CAD build for the part. Positions are in the model's coordinates, mm. Round coordinates to 2 decimals unless told otherwise and drop trailing zeros. Order: outer loops, then holes, each group sorted by start corner. A loop starts at its lowest first (then second) coordinate and runs counter-clockwise, first axis right, second up. Notation, with made-up numbers: (-34.75, 14.5) - (-5.75, 14.5) arc R24 cw to (-5.75, 28.5) - close; hole circle Ø8 at (39, 39). An arc over 180 degrees is marked (long way). Use one line per item in the form item = value. Start each with the question number.
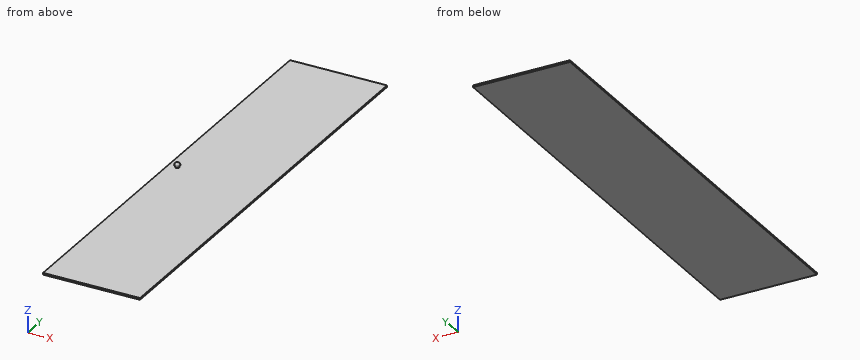
from build123d import *

# Parameters (mm, degrees)
SKETCH1_W           = 550
SKETCH1_H           = 2550
BOSS_EXTRUDE1_DEPTH = 10
SKETCH2_R           = 10
BOSS_EXTRUDE2_DEPTH = 10
SKETCH3_R           = 15
BOSS_EXTRUDE3_DEPTH = 15
FILLET1_R           = 10


with BuildPart() as part:
    # Sketch1 → Boss-Extrude1 (new body)
    with BuildSketch(Plane.XY):
        Rectangle(SKETCH1_W, SKETCH1_H)
    extrude(amount=BOSS_EXTRUDE1_DEPTH)

    # Sketch2 → Boss-Extrude2 (add)
    with BuildSketch(Plane.XY.offset(10)):
        with Locations((-225, 20)):
            Circle(SKETCH2_R)
    extrude(amount=BOSS_EXTRUDE2_DEPTH)

    # Sketch3 → Boss-Extrude3 (add)
    with BuildSketch(Plane.XY.offset(20)):
        with Locations((-225, 20)):
            Circle(SKETCH3_R)
    extrude(amount=BOSS_EXTRUDE3_DEPTH)

    # Fillet1
    fillet1_edges = [part.edges().sort_by_distance(p)[0] for p in [
        (-240, 20, 35),
    ]]
    fillet(fillet1_edges, radius=FILLET1_R)


solid = part.part
(1) Flat gauge pin, fed straight in: P1, Ø4, axis at x = -50, y = 576.5, coming from the +Z side. Where does the tip first touch, or does it go through?
(2) Slice it at A-A (x = 127). Give the cut face in (y, z).
(3) Slice it at B-B (y = -773.5). Give the cut face in (x, z), and give its area (3 significant figures).
(4) Wall check: line 1 (Z direction, x = -113, y = 231); line 2 (X direction, y = 12.5, z = 23.5); line 3 (Y direction, x = -215, z = 22). Give the ranges that are in metal, low to high. Write a range as [from, to].
Results list:
q1.P1 = 10
q2.outline = (-1275, 0) - (1275, 0) - (1275, 10) - (-1275, 10) - close
q3.outline = (-275, 0) - (275, 0) - (275, 10) - (-275, 10) - close
q3.area = 5,500 mm²
q4.line_1 = [0, 10]
q4.line_2 = [-237.99, -212.01]
q4.line_3 = [8.82, 31.18]
